from build123d import *

# Parameters (mm, degrees)
SKETCH1_R           = 30
SKETCH1_R_2         = 1
SKETCH1_R_3         = 4.9
BOSS_EXTRUDE1_DEPTH = 7.46
SKETCH3_W           = 7.46
SKETCH3_H           = 44.5
BOSS_EXTRUDE2_DEPTH = 60.3
SKETCH4_R           = 1
SKETCH4_W           = 19.5
SKETCH4_H           = 40.3
CUT_EXTRUDE2_DEPTH  = 85.690126933
SKETCH5_R           = 10.6
CUT_EXTRUDE3_DEPTH  = 4.96
SKETCH6_W           = 19.5
SKETCH6_H           = 54
CUT_EXTRUDE4_DEPTH  = 3
SKETCH7_W           = 2
SKETCH7_H           = 6.85
CUT_EXTRUDE5_DEPTH  = 2.5
SKETCH8_R           = 2.75
CUT_EXTRUDE6_DEPTH  = 85.690126933


with BuildPart() as part:
    # Sketch1 → Boss-Extrude1 (new body)
    with BuildSketch(Plane(origin=(0, 0, 0), x_dir=(1, 0, 0), z_dir=(0, 1, 0))):
        with Locations(Location((0, 0, 0), (0, 0, 90))):
            Circle(SKETCH1_R)
        with Locations(Location((7, 0, 0), (0, 0, 90))):
            Circle(SKETCH1_R_2, mode=Mode.SUBTRACT)
        with Locations(Location((0, -7, 0), (0, 0, 90))):
            Circle(SKETCH1_R_2, mode=Mode.SUBTRACT)
        with Locations(Location((-7, 0, 0), (0, 0, 90))):
            Circle(SKETCH1_R_2, mode=Mode.SUBTRACT)
        with Locations(Location((0, 7, 0), (0, 0, 90))):
            Circle(SKETCH1_R_2, mode=Mode.SUBTRACT)
        with Locations(Location((0, 0, 0), (0, 0, 90))):
            Circle(SKETCH1_R_3, mode=Mode.SUBTRACT)
    extrude(amount=BOSS_EXTRUDE1_DEPTH)

    # Sketch3 → Boss-Extrude2 (add)
    with BuildSketch(Plane(origin=(0, 7.46, 0), x_dir=(1, 0, 0), z_dir=(0, 1, 0))):
        with Locations((14.73, 0)):
            Rectangle(SKETCH3_W, SKETCH3_H)
    extrude(amount=BOSS_EXTRUDE2_DEPTH)

    # Sketch4 → Cut-Extrude2 (cut, through all)
    with BuildSketch(Plane.ZY.offset(-11)):
        with Locations((-5, 61.93)):
            Circle(SKETCH4_R)
        with Locations((5, 61.93)):
            Circle(SKETCH4_R)
        with Locations((5, 13.29)):
            Circle(SKETCH4_R)
        with Locations((-5, 13.29)):
            Circle(SKETCH4_R)
        with Locations((0, 37.61)):
            Rectangle(SKETCH4_W, SKETCH4_H)
    extrude(amount=-CUT_EXTRUDE2_DEPTH, mode=Mode.SUBTRACT)

    # Sketch5 → Cut-Extrude3 (cut)
    with BuildSketch(Plane(origin=(0, 7.46, 0), x_dir=(1, 0, 0), z_dir=(0, 1, 0))):
        with Locations(Location((0, 0, 0), (0, 0, 270))):
            Circle(SKETCH5_R)
    extrude(amount=-CUT_EXTRUDE3_DEPTH, mode=Mode.SUBTRACT)

    # Sketch6 → Cut-Extrude4 (cut)
    with BuildSketch(Plane.ZY.offset(-11)):
        with Locations((0, 37.61)):
            Rectangle(SKETCH6_W, SKETCH6_H)
    extrude(amount=-CUT_EXTRUDE4_DEPTH, mode=Mode.SUBTRACT)

    # Sketch7 → Cut-Extrude5 (cut)
    with BuildSketch(Plane.ZY.offset(-14)):
        with Locations((0, 61.185)):
            Rectangle(SKETCH7_W, SKETCH7_H)
        with Locations((0, 14.035)):
            Rectangle(SKETCH7_W, SKETCH7_H)
    extrude(amount=-CUT_EXTRUDE5_DEPTH, mode=Mode.SUBTRACT)

    # Sketch8 → Cut-Extrude6 (cut, through all)
    with BuildSketch(Plane.ZY.offset(-11)):
        with Locations((-16, 37.61)):
            Circle(SKETCH8_R)
        with Locations((-16, 45.61)):
            Circle(SKETCH8_R)
        with Locations((-16, 53.61)):
            Circle(SKETCH8_R)
        with Locations((-16, 61.61)):
            Circle(SKETCH8_R)
        with Locations((-16, 13.61)):
            Circle(SKETCH8_R)
        with Locations((-16, 21.61)):
            Circle(SKETCH8_R)
        with Locations((-16, 29.61)):
            Circle(SKETCH8_R)
        with Locations((16, 29.61)):
            Circle(SKETCH8_R)
        with Locations((16, 21.61)):
            Circle(SKETCH8_R)
        with Locations((16, 13.61)):
            Circle(SKETCH8_R)
        with Locations((16, 61.61)):
            Circle(SKETCH8_R)
        with Locations((16, 53.61)):
            Circle(SKETCH8_R)
        with Locations((16, 45.61)):
            Circle(SKETCH8_R)
        with Locations((16, 37.61)):
            Circle(SKETCH8_R)
    extrude(amount=-CUT_EXTRUDE6_DEPTH, mode=Mode.SUBTRACT)


solid = part.part
Geometry: final body of the model. Coordinates: model frame, mm. A direction names the side the tool comes from. Give positions to 0.01 mm unless a question says otherwise; leave off trailing zeros. Loops run counter-clockwise (first coordinate to the right, second up) from the corner with the lowest first, then second, coordinate; pieces in that order, holes last. Notation, with made-up numbers: (43.5, -32.75) - (59.5, -32.75) arc R25 cw to (59.5, -13.75) - close; hole circle Ø10 at (39, 69). An arc over 180 degrees is marked (long way). Answer as CSV lines item,"result". Start each with the question number.
1. Ray query, L1, parallel to Y at x = 15.5, z = -5; L2, parallel to Z at x = 12.5, y = 31; L3, parallel to Z at x = 14, y = 37. Return the intervals inside material, ascending.
2. Section B-B, the plane z = 0. Give the number of separate pieces and of enclosed holes in the cut face, plus the area to 3 significant figures.
3. Section C-C, the plane x = 2.5. Return loops of the section in (y, z), plus the area to 3 significant figures.
4. Reachability of faces 1 (the face through (11, 37, 10)), 2 (the face through (-6.45, 5.01, -8.41)), 3 (the face through (12, 64.61, 0)) from +Z, -Z, +X, -X, +Y, -Y: full face, straight path, thin tool, end or side. Return the list, or none.
5. Pin query (flat end, axial travel): P1, Ø4, axis at x = -2.5, z = -23.5, coming from the +Y side; P2, Ø3.5, axis at y = 59.5, z = -7.5, coming from the -X side; P3, Ø9, axis at y = 29.61, z = 16, coming from the -X side. Return the tip coordinate at first contact, or that it passes through.
6. Section D-D, the plane z = 7. Return loops of the section in (x, y).
7. Section A-A, the plane y = 21.61. Return loops of the section in (x, z).
8. Draft query along X for faces 4 (the face through (-1.32, 3.68, 29.97)), 5 (the face through (14.678, 56.337, 15.642)), 6 (the face through (-8, 1, 0)). Return one class per face: released by +X, released by -X, zero draft, split by the parting line, or undercut.
Answers:
1,L1,"y = 0 to 12.29, 14.29 to 17.46, 57.76 to 60.93, 62.93 to 67.76"
1,L2,"z = -22.25 to -18.37, -13.63 to -9.75, 9.75 to 13.63, 18.37 to 22.25"
1,L3,"z = -22.25 to -18.68, -13.32 to -9.75, 9.75 to 13.32, 18.68 to 22.25"
2,separate pieces,"5"
2,enclosed holes,"0"
2,area,"382 mm2"
3,outline,"(0, -29.9) - (7.46, -29.9) - (7.46, -10.3) - (2.5, -10.3) - (2.5, -4.21) - (0, -4.21) - close; (0, 4.21) - (2.5, 4.21) - (2.5, 10.3) - (7.46, 10.3) - (7.46, 29.9) - (0, 29.9) - close"
3,area,"323 mm2"
4,face 1,"+Z, -Z, -X, +Y"
4,face 2,"+Y"
4,face 3,"-X"
5,P1,"stops at y = 7.46"
5,P2,"stops at x = 14"
5,P3,"stops at x = 11"
6,outline,"(-29.17, 0) - (-1, 0) - (-1, 2.5) - (-7.96, 2.5) - (-7.96, 7.46) - (-29.17, 7.46) - close; (1, 0) - (29.17, 0) - (29.17, 7.46) - (18.46, 7.46) - (18.46, 17.46) - (14, 17.46) - (14, 10.61) - (11, 10.61) - (11, 7.46) - (7.96, 7.46) - (7.96, 2.5) - (1, 2.5) - close; (11, 64.61) - (14, 64.61) - (14, 57.76) - (18.46, 57.76) - (18.46, 67.76) - (11, 67.76) - close"
7,outline,"(11, -22.25) - (18.46, -22.25) - (18.46, -18.75) - (11, -18.75) - close; (11, -13.25) - (18.46, -13.25) - (18.46, -9.75) - (11, -9.75) - close; (11, 9.75) - (18.46, 9.75) - (18.46, 13.25) - (11, 13.25) - close; (11, 18.75) - (18.46, 18.75) - (18.46, 22.25) - (11, 22.25) - close"
8,face 4,"split by the parting line"
8,face 5,"zero draft"
8,face 6,"undercut"
